from build123d import *

# Parameters (mm, degrees)
SKETCH1_W           = 134.8
SKETCH1_H           = 12.7
SKETCH1_R           = 1.8288
BOSS_EXTRUDE1_DEPTH = 1.5875
SKETCH2_R           = 1.8288
CUT_EXTRUDE1_DEPTH  = 137.401796749


with BuildPart() as part:
    # Sketch1 → Boss-Extrude1 (new body)
    with BuildSketch(Plane(origin=(0, 0, 0), x_dir=(1, 0, 0), z_dir=(0, 1, 0))):
        with Locations((68.4, 6.35)):
            Rectangle(SKETCH1_W, SKETCH1_H)
        with Locations(Location((6, 6.35, 0), (0, 0, 270))):
            Circle(SKETCH1_R, mode=Mode.SUBTRACT)
        with Locations(Location((130.8, 6.35, 0), (0, 0, 270))):
            Circle(SKETCH1_R, mode=Mode.SUBTRACT)
    extrude(amount=BOSS_EXTRUDE1_DEPTH)

    # Sketch2 → Cut-Extrude1 (cut, through all)
    with BuildSketch(Plane(origin=(0, 1.5875, 0), x_dir=(1, 0, 0), z_dir=(0, 1, 0))):
        with Locations(Location((26.8, 6.35, 0), (0, 0, 270))):
            Circle(SKETCH2_R)
        with Locations(Location((47.6, 6.35, 0), (0, 0, 270))):
            Circle(SKETCH2_R)
        with Locations(Location((68.4, 6.35, 0), (0, 0, 270))):
            Circle(SKETCH2_R)
        with Locations(Location((89.2, 6.35, 0), (0, 0, 270))):
            Circle(SKETCH2_R)
        with Locations(Location((110, 6.35, 0), (0, 0, 270))):
            Circle(SKETCH2_R)
    extrude(amount=-CUT_EXTRUDE1_DEPTH, mode=Mode.SUBTRACT)


solid = part.part
Design review of the part built by this model. Coordinates are the model's own, in mm. Give positions to 0.01 mm unless a question says otherwise; leave off trailing zeros. Loops run counter-clockwise (first coordinate to the right, second up) from the corner with the lowest first, then second, coordinate; pieces in that order, holes last. Notation, with made-up numbers: (-31, 49) - (6, 49) arc R10 cw to (6, 57) - close; hole circle Ø9 at (23.25, 0.25). An arc over 180 degrees is marked (long way). Use CSV: the item, a comma, the result in double quotes. Start each with the question number.
1. Add section B-B (z = -6.35). Count the separate pieces of the cut face and the enclosed holes in it, plus the area to 3 significant figures.
2. Insertion check: P1, Ø2, axis at x = 47.6, z = -6.35, coming from the +Y side; P2, Ø5, axis at x = 89.2, z = -6.35, coming from the +Y side. Each pin has a flat end and moves straight along its axis. Give the tip position at first contact, or say it passes through.
3. Add section A-A (x = 6). State the section outline as (y, z) points.
4. Wall thickness on L1, parallel to Z at x = 26, y = 0.75; L2, parallel to Z at x = 28, y = 0.1: over which ranges is each line inside the solid? List them lowest first.
5. Add section C-C (y = 0.4). State the section outline as (x, z) points, plus the area to 3 significant figures.
6. Draft analysis for pull direction X (two halves, no side actions). For faces 1 (the cylindrical face through (90.742, 0.805, -5.367)), 2 (the flat face through (67, 0, -4)), state which applies: released by +X, released by -X, zero draft, split by the parting line, or undercut.
Results found:
1,separate pieces,"8"
1,enclosed holes,"0"
1,area,"173 mm²"
2,P1,"passes through"
2,P2,"stops at y = 1.59"
3,outline,"(0, -12.7) - (1.59, -12.7) - (1.59, -8.18) - (0, -8.18) - close; (0, -4.52) - (1.59, -4.52) - (1.59, 0) - (0, 0) - close"
4,L1,"z = -12.7 to -7.99, -4.71 to 0"
4,L2,"z = -12.7 to -7.73, -4.97 to 0"
5,outline,"(1, -12.7) - (135.8, -12.7) - (135.8, 0) - (1, 0) - close; hole circle Ø3.66 at (6, -6.35); hole circle Ø3.66 at (26.8, -6.35); hole circle Ø3.66 at (47.6, -6.35); hole circle Ø3.66 at (68.4, -6.35); hole circle Ø3.66 at (89.2, -6.35); hole circle Ø3.66 at (110, -6.35); hole circle Ø3.66 at (130.8, -6.35)"
5,area,"1,640 mm²"
6,face 1,"undercut"
6,face 2,"zero draft"
